from build123d import *

# Parameters (mm, degrees)
F1_DEPTH = 17
F2_R     = 1.65
F3_DEPTH = 40.001
F5_DEPTH = 15.001


with BuildPart() as f1:
    # F0 (on Front) → F1 (new body, symmetric)
    with BuildSketch(Plane.XZ):
        with BuildLine():
            Line((15, 0), (2, 0))
            ThreePointArc((2, 0), (0.585786, -0.585786), (0, -2))
            Line((0, -2), (0, -40))
            Line((0, -40), (1.5, -40))
            Line((1.5, -40), (1.5, -2))
            ThreePointArc((1.5, -2), (1.646447, -1.646447), (2, -1.5))
            Line((2, -1.5), (15, -1.5))
            Line((15, -1.5), (15, 0))
        make_face()
    extrude(amount=F1_DEPTH, both=True)

    # F2 (on Top) → F3 (cut, through all)
    with BuildSketch(Plane.XY):
        with BuildLine():
            ThreePointArc((12.194882, -14.160663), (13.638451, -12.327331), (11.805118, -10.883762))
            ThreePointArc((11.805118, -10.883762), (8.495594, -11.044643), (5.195887, -10.743362))
            ThreePointArc((5.195887, -10.743362), (3.302904, -12.107773), (4.667315, -14.000755))
            ThreePointArc((4.667315, -14.000755), (8.425508, -14.343899), (12.194882, -14.160663))
        make_face()
        with Locations((9, 12.7)):
            Circle(F2_R)
    extrude(amount=-F3_DEPTH, mode=Mode.SUBTRACT)

    # F4 (on Right) → F5 (cut, through all)
    with BuildSketch(Plane.YZ):
        with BuildLine():
            ThreePointArc((11.05, -34), (12.7, -35.65), (14.35, -34))
            Line((14.35, -34), (14.35, -12))
            ThreePointArc((14.35, -12), (12.7, -10.35), (11.05, -12))
            Line((11.05, -12), (11.05, -34))
        make_face()
        with BuildLine():
            ThreePointArc((-14.35, -34), (-12.7, -35.65), (-11.05, -34))
            Line((-11.05, -34), (-11.05, -12))
            ThreePointArc((-11.05, -12), (-12.7, -10.35), (-14.35, -12))
            Line((-14.35, -12), (-14.35, -34))
        make_face()
    extrude(amount=F5_DEPTH, mode=Mode.SUBTRACT)


solid = f1.part
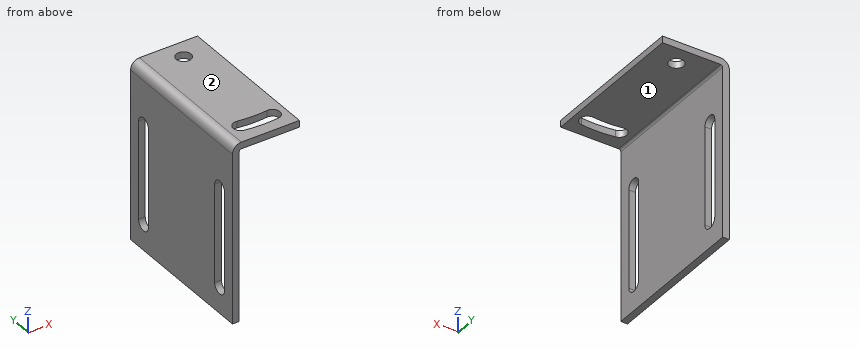
The model under review builds one solid part; all positions refer to its coordinate system, in mm. Face numbers are marked on the shaded views. A direction names the side the tool comes from. Coordinates: 2 decimals unless noted, no trailing zeros. Write each loop counter-clockwise with the first axis right and the second up, starting at its lowest first coordinate (ties: lowest second). Pieces come first, ordered by that corner, then holes. Notation, with made-up numbers: (-1.5, -13.5) - (11.5, -13.5) arc R33 ccw to (11.5, 25.5) - close; hole circle Ø9 at (6, -37). An arc over 180 degrees is marked (long way). Answer as CSV lines item,"result".
(1) Clearance check with flat-ended pins moving along their axes: pin 1 Ø10 at (y, z) = (-10.5, -35.5) entering from +X; pin 2 Ø2 at (x, y) = (12, -4) entering from +Z; pin 3 Ø1.5 at (x, y) = (9.5, 6.5) entering from -Z. State where each tip first meets the part, or that it passes through.
Data:
pin 1,"stops at x = 1.5"
pin 2,"stops at z = 0"
pin 3,"stops at z = -1.5"
(2) We need section B-B (x = 9). Give the boundary of the cut face in (y, z), plus the area to 3 significant figures.
Data:
outline,"(-17, -1.5) - (-14.35, -1.5) - (-14.35, 0) - (-17, 0) - close; (-11.05, -1.5) - (11.05, -1.5) - (11.05, 0) - (-11.05, 0) - close; (14.35, -1.5) - (17, -1.5) - (17, 0) - (14.35, 0) - close"
area,"41.1 mm2"
(3) For line 1 along Y through (x, z) = (9, -1.15); line 2 along Z through (x, y) = (13.75, 9); line 3 along X through (y, z) = (-3, -10), list the stretches that pass through material, from the lowest coordinate up. Write a range as [from, to].
Data:
line 1,"y = [-17, -14.35], [-11.05, 11.05], [14.35, 17]"
line 2,"z = [-1.5, 0]"
line 3,"x = [0, 1.5]"
(4) We need section D-D (y = -4). Give the boundary of the cut face in (x, z), plus the area to 3 significant figures.
Data:
outline,"(0, -40) - (1.5, -40) - (1.5, -2) arc R0.5 cw to (2, -1.5) - (15, -1.5) - (15, 0) - (2, 0) arc R2 ccw to (0, -2) - close"
area,"79.4 mm2"
(5) We need section A-A (z = -29). Give the boundary of the cut face in (x, y).
Data:
outline,"(0, -17) - (1.5, -17) - (1.5, -14.35) - (0, -14.35) - close; (0, -11.05) - (1.5, -11.05) - (1.5, 11.05) - (0, 11.05) - close; (0, 14.35) - (1.5, 14.35) - (1.5, 17) - (0, 17) - close"
(6) We need section C-C (y = 12.7). Give the boundary of the cut face in (x, z), plus the area to 3 significant figures.
Data:
outline,"(0, -40) - (1.5, -40) - (1.5, -35.65) - (0, -35.65) - close; (0, -10.35) - (1.5, -10.35) - (1.5, -2) arc R0.5 cw to (2, -1.5) - (7.35, -1.5) - (7.35, 0) - (2, 0) arc R2 ccw to (0, -2) - close; (10.65, -1.5) - (15, -1.5) - (15, 0) - (10.65, 0) - close"
area,"36.5 mm2"
(7) Tool access review of the marked faces 1 and 2: name each direction out of +Z, -Z, +X, -X, +Y, -Y from which nothing blocks a thin tool from reaching the whole face with its end or side.
Data:
face 1,"-Z, +X, +Y, -Y"
face 2,"+Z, +X, -X, +Y, -Y"
